The listing builds one solid part. Answer for the finished solid, in the listing's coordinates (mm). Face numbers are marked on the shaded views. A direction names the side the tool comes from. Coordinates: 2 decimals unless noted, no trailing zeros. Write each loop counter-clockwise with the first axis right and the second up, starting at its lowest first coordinate (ties: lowest second). Pieces come first, ordered by that corner, then holes.
from build123d import *

# Parameters (mm, degrees)
SKETCH_3_R      = 2
EXTRUDE_1_DEPTH = 4


with BuildPart() as part:
    # 草图3 → 凸台-拉伸1 (new body)
    with BuildSketch(Plane.XY):
        with BuildLine():
            Line((-37.667405861, 56.89708202), (-46.686841808, 58.42631375))
            ThreePointArc((-46.686841808, 58.42631375), (-33.287089683, 19.828920451), (5.267276505, 6.30586701))
            Line((5.267276505, 6.30586701), (4.265537779, 15.188089459))
            Line((4.265537779, 15.188089459), (0, 17.509783315))
            Line((0, 17.509783315), (-4.788956139, 15.257523407))
            ThreePointArc((-4.788956139, 15.257523407), (-27.767557087, 26.988061571), (-37.98334573, 50.67897311))
            Line((-37.98334573, 50.67897311), (-35.5, 53.009783315))
            Line((-35.5, 53.009783315), (-37.667405861, 56.89708202))
        make_face()
        with Locations((0, 10.509783315)):
            Circle(SKETCH_3_R, mode=Mode.SUBTRACT)
        with Locations((-30.0520382, 22.957745114)):
            Circle(SKETCH_3_R, mode=Mode.SUBTRACT)
        with Locations((-42.5, 53.009783315)):
            Circle(SKETCH_3_R, mode=Mode.SUBTRACT)
    extrude(amount=EXTRUDE_1_DEPTH)


solid = part.part
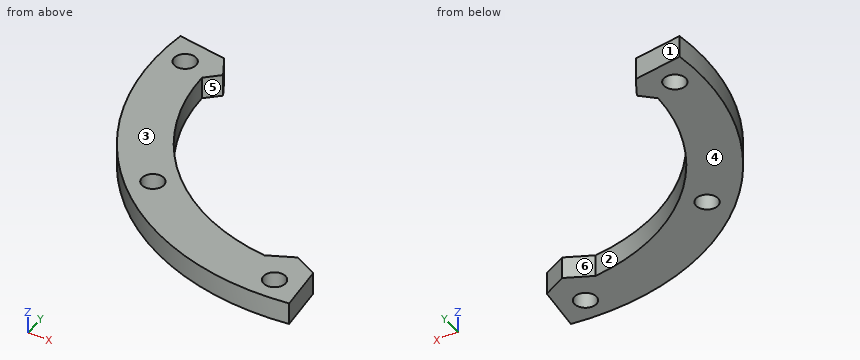
Q1. Given pin 1 (2 mm diameter, centred on x = -15.5, z = 1, fed in from -Y), flat-ended and moving along its own axis, determine where the tip first touches the part or whether it passes through.
Answers below:
pin 1: stops at y = 8.3
Q2. Find the intervals of material crossed by probe 1 along Y at (x, z) = (0, 2.75); probe 2 along X at (y, z) = (53, 2.15); probe 3 along Y at (x, z) = (-28.5, 3.4), in increasing order.
Answers below:
probe 1: y = 6.01 to 8.51, 12.51 to 17.51
probe 2: x = -47 to -44.5, -40.5 to -35.51
probe 3: y = 15.64 to 21.7, 24.22 to 27.79
Q3. The part is cut by section B-B, the plane z = 2.4. Write down the section's boundary in (x, y).
Answers below:
outline: (-46.69, 58.43) arc R47 ccw to (5.27, 6.31) - (4.27, 15.19) - (0, 17.51) - (-4.79, 15.26) arc R38.05 cw to (-37.98, 50.68) - (-35.5, 53.01) - (-37.67, 56.9) - close; hole circle Ø4 at (-42.5, 53.01); hole circle Ø4 at (-30.05, 22.96); hole circle Ø4 at (0, 10.51)
Q4. Determine the mould class of the marked faces 1, 2 and 3 for opening direction Y: released by +Y, released by -Y, zero draft, split by the parting line, or undercut.
Answers below:
face 1: released by +Y
face 2: undercut
face 3: zero draft
Q5. The part is cut by section A-A, the plane x = -42.5. Write down the section's boundary in (y, z).
Answers below:
outline: (32.94, 0) - (51.01, 0) - (51.01, 4) - (32.94, 4) - close; (55.01, 0) - (57.72, 0) - (57.72, 4) - (55.01, 4) - close
Q6. Which of the six approach directions +Z, -Z, +X, -X, +Y, -Y give full straight-line access (tool end or side, diameter ignored) to the marked faces 4, 5 and 6?
Answers below:
face 4: -Z, +X, -X, +Y, -Y
face 5: +Z, -Z, +X
face 6: +Z, -Z, +Y
Q7. The part is cut by section C-C, the plane x = -13. Write down the section's boundary in (y, z), then the cut area to 3 significant figures.
Answers below:
outline: (7.84, 0) - (17.24, 0) - (17.24, 4) - (7.84, 4) - close
area: 37.6 mm2
Q8. The part is cut by section D-D, the plane y = 38.5. Write down the section's boundary in (x, z), then the cut area to 3 significant figures.
Answers below:
outline: (-44.7, 0) - (-35.18, 0) - (-35.18, 4) - (-44.7, 4) - close
area: 38.1 mm2
